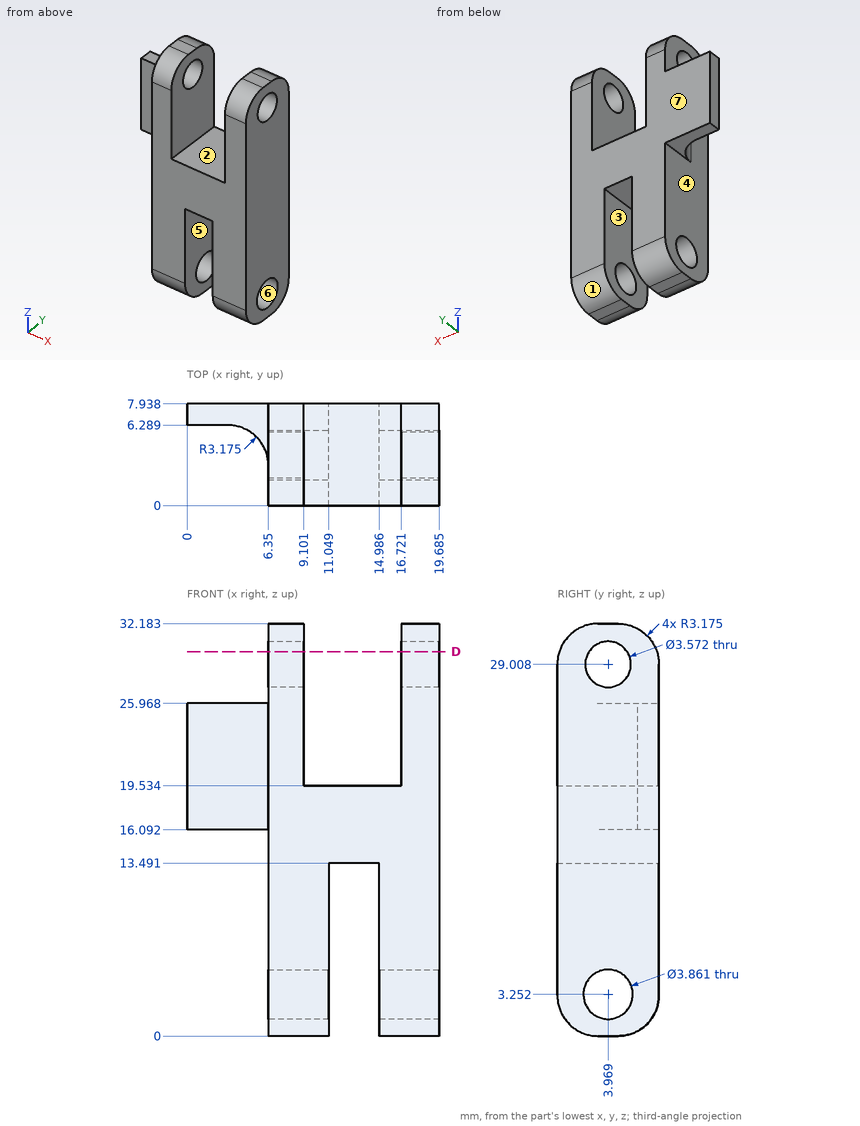
For this review, use the dimensioned drawing (mm, ordinates from the lowest corner) and the shaded views. A direction names the side the tool comes from. Round coordinates to 2 decimals unless told otherwise and drop trailing zeros. One line per item, written item: value. Start each with the question number.
Q1. Machinability: for the marked faces 1, 2, 3 and 4, which of the approach directions +Z, -Z, +X, -X, +Y, -Y give a long, thin tool a straight path to every point of the face, cutting with its end or side? Answer none if there is none.
Q2. Clearance check with flat-ended pins moving along their axes: pin 1 Ø3 at (x, z) = (4, 8) entering from +Y; pin 2 Ø2.5 at (y, z) = (4, 26.5) entering from -X; pin 3 Ø1.6 at (x, z) = (1, 23) entering from -Y; pin 4 Ø3 at (x, y) = (4.5, 6.5) entering from -Z. State where each tip first meets the part, or that it passes through.
Q3. Mouldability with a two-part tool opening along Y and no side actions: class the marked faces 5, 6 and 7 as released by +Y, released by -Y, zero draft, split by the parting line, or undercut.
Q4. Take a section at D-D (z = 30). Count the separate pieces of the cut face and the enclosed holes in it.
Q5. Wall thickness on line 1 (Z direction, x = 6.5, y = 3) (1 decimal); line 2 (X direction, y = 7.75, z = 23.5) (1 decimal); line 3 (Y direction, x = 6.5, z = 29) (1 decimal): over which ranges is each line inside the solid? List them lowest first.
Reported:
1. face 1: -Z, +X, -X, +Y
1. face 2: +Z, +Y, -Y
1. face 3: -Z, +Y, -Y
1. face 4: -X, -Y
2. pin 1: passes through
2. pin 2: stops at x = 5.63
2. pin 3: stops at y = 6.29
2. pin 4: stops at z = 16.09
3. face 5: zero draft
3. face 6: undercut
3. face 7: released by +Y
4. separate pieces: 4
4. enclosed holes: 0
5. line 1: z = 0 to 1.6, 4.9 to 27.5, 30.5 to 32.2
5. line 2: x = 0 to 9.1, 16.7 to 19.7
5. line 3: y = 0 to 2.2, 5.8 to 7.9
